from build123d import *

# Parameters (mm, degrees)
SKETCH1_R           = 19.05
SKETCH1_R_2         = 10.9873
BOSS_EXTRUDE1_DEPTH = 6.35
SKETCH2_R           = 21.59
SKETCH2_R_2         = 10.9873
BOSS_EXTRUDE2_DEPTH = 2.54
SKETCH3_R           = 10.9873
SKETCH3_R_2         = 7.9375
BOSS_EXTRUDE3_DEPTH = 2.794
CHAMFER1_SIZE       = 0.635
CHAMFER2_SIZE       = 0.635


with BuildPart() as part:
    # Sketch1 → Boss-Extrude1 (new body, symmetric)
    with BuildSketch(Plane.XY):
        Circle(SKETCH1_R)
        Circle(SKETCH1_R_2, mode=Mode.SUBTRACT)
    extrude(amount=BOSS_EXTRUDE1_DEPTH, both=True)

    # Sketch2 → Boss-Extrude2 (add, symmetric)
    with BuildSketch(Plane.XY):
        Circle(SKETCH2_R)
        Circle(SKETCH2_R_2, mode=Mode.SUBTRACT)
    extrude(amount=BOSS_EXTRUDE2_DEPTH, both=True)

    # Sketch3 → Boss-Extrude3 (add)
    with BuildSketch(Plane.XY.offset(6.35)):
        Circle(SKETCH3_R)
        Circle(SKETCH3_R_2, mode=Mode.SUBTRACT)
    extrude(amount=-BOSS_EXTRUDE3_DEPTH)

    # Chamfer1
    chamfer1_edges = [part.edges().sort_by_distance(p)[0] for p in [
        (-21.59, 0, 2.54),
        (-21.59, 0, -2.54),
        (-19.05, 0, -6.35),
        (-19.05, 0, 6.35),
    ]]
    chamfer(chamfer1_edges, length=CHAMFER1_SIZE)

    # Chamfer2
    chamfer2_edges = [part.edges().sort_by_distance(p)[0] for p in [
        (-10.9873, 0, -6.35),
    ]]
    chamfer(chamfer2_edges, length=CHAMFER2_SIZE)


solid = part.part
For this review, take the finished solid that the model builds, in its own axes (mm). A direction names the side the tool comes from. Round coordinates to 2 decimals unless told otherwise and drop trailing zeros. Loops run counter-clockwise (first coordinate to the right, second up) from the corner with the lowest first, then second, coordinate; pieces in that order, holes last. Notation, with made-up numbers: (75.25, 89) - (130.25, 89) arc R25 ccw to (130.25, 113) - close; hole circle Ø3 at (8.25, -24.75). An arc over 180 degrees is marked (long way). Use one line per item in the form item = value.
Item 1: Consider section D-D on z = 0. Write out the cut boundary in (x, y).
Answers:
outline = circle Ø43.18 at (0, 0); hole circle Ø21.97 at (0, 0)
Item 2: Clearance check with flat-ended pins moving along their axes: P1, Ø13, axis at x = 0, y = 0, coming from the +Z side; P2, Ø6, axis at y = -5, z = 2.5, coming from the -X side; P3, Ø3, axis at x = 16, z = 5, coming from the +Y side; P4, Ø11, axis at x = -4.5, y = 3.5, coming from the -Z side. State where each tip first meets the part, or that it passes through.
Answers:
P1 = through
P2 = -21.49
P3 = 12.36
P4 = -5.93
Item 3: Tool access review of faces 1 (the flat face through (6, 6, 3.556)), 2 (the flat face through (0, -12, -6.35)), 3 (the cylindrical face through (-15.12, -11.59, 4.15)): name each direction out of +Z, -Z, +X, -X, +Y, -Y from which nothing blocks a thin tool from reaching the whole face with its end or side.
Answers:
face_1 = -Z
face_2 = -Z, +X, -X, +Y, -Y
face_3 = +Z
Item 4: Consider section C-C on z = -4.5. Write out the cut boundary in (x, y), then the cut area to 3 significant figures.
Answers:
outline = circle Ø38.1 at (0, 0); hole circle Ø21.97 at (0, 0)
area = 761 mm^2
Item 5: For line 1 (Y direction, x = 0, z = 5.3); line 2 (Y direction, x = 0, z = -0.25); line 3 (Z direction, x = 18, y = -9), list the stretches that pass through material, from the lowest coordinate up.
Answers:
line_1 = -19.05 to -7.94, 7.94 to 19.05
line_2 = -21.59 to -10.99, 10.99 to 21.59
line_3 = -2.54 to 2.54
Item 6: Mouldability with a two-part tool opening along X and no side actions: class faces 4 (the cylindrical face through (-15.913, 14.592, 0.027)), 5 (the flat face through (8, -4, 6.35)), 6 (the cylindrical face through (10.48, 3.3, -1.14)) as +X half, -X half, draft (parallel to the pull), parting line (faces both ways), or undercut.
Answers:
face_4 = parting line
face_5 = draft
face_6 = undercut
